The listing builds one solid part. Answer for the finished solid, in the listing's coordinates (mm). A direction names the side the tool comes from. Give positions to 0.01 mm unless a question says otherwise; leave off trailing zeros. Write each loop counter-clockwise with the first axis right and the second up, starting at its lowest first coordinate (ties: lowest second). Pieces come first, ordered by that corner, then holes. Notation, with made-up numbers: (24.25, -8.75) -> (57.25, -8.75) arc R9 ccw to (57.25, 2.25) -> close; hole circle Ø10 at (20, 31). An arc over 180 degrees is marked (long way). Put each result on its own line as item: value. Start each with the question number.
1) Flat-ended cylindrical pins translate along their axes: pin 1 Ø3.5 at (x, z) = (20.07, -1.25) entering from -Y; pin 2 Ø1.8 at (x, z) = (-8.86, -1.25) entering from +Y; pin 3 Ø7.5 at (x, y) = (11, 8) entering from +Z; pin 4 Ø1.1 at (y, z) = (13.5, 14) entering from +X. Find the tip coordinate at first contact, or state that the pin passes through.
2) A cutting plane is placed at A-A (z = 1). Write down the section's boundary in (x, y), then the cut area to 3 significant figures.
3) A cutting plane is placed at D-D (x = -11). Write down the section's boundary in (y, z).
4) Find the intervals of material crossed by line 1 along Z through (x, y) = (13.5, 10.75); line 2 along X through (y, z) = (6.5, 3); line 3 along Z through (x, y) = (20.5, 11.75), in increasing order. Write a range as from..to.
5) A cutting plane is placed at B-B (x = -1). Write down the section's boundary in (y, z).
6) For a pull along Z with two mould halves and no side action, classify faces 4 (the flat face through (6, 0, -9)), 5 (the flat face through (6, 7, 4.75)), 6 (the cylindrical face through (-7.93, 14.01, -0.66)), 7 (the flat face through (6, 8, -12.536)) as released by +Z, released by -Z, zero draft, split by the parting line, or undercut.
7) A cutting plane is placed at C-C (y = 10). Write down the section's boundary in (x, z), then the cut area to 3 significant figures.
8) For faces 1 (the flat face through (6, 7, -7.25)), 2 (the flat face through (-13, 12, 2.464)), 3 (the flat face through (-11.714, 13, -15)), determine the directions among +Z, -Z, +X, -X, +Y, -Y from which every point of the face is accessible in a straight line to the end or side of a thin tool.
from build123d import *

# Parameters (mm, degrees)
ESQUISSE1_W             = 34.285714285
ESQUISSE1_H             = 23
ESQUISSE1_W_2           = 25
ESQUISSE1_H_2           = 12
BOSS_EXTRU_1_DEPTH      = 15
ESQUISSE2_W             = 7
ESQUISSE2_H             = 8
ENL_V_MAT_EXTRU_1_DEPTH = 60
ESQUISSE3_R             = 1.1
ENL_V_MAT_EXTRU_2_DEPTH = 10
ESQUISSE4_W             = 7
ESQUISSE4_H             = 8
BOSS_EXTRU_2_DEPTH      = 20
ESQUISSE7_W             = 23
ESQUISSE7_H             = 11.477873567
ENL_V_MAT_EXTRU_3_DEPTH = 20
ESQUISSE6_R             = 1
ENL_V_MAT_EXTRU_4_DEPTH = 20


with BuildPart() as part:
    # Esquisse1 → Boss.-Extru.1 (new body)
    with BuildSketch(Plane(origin=(0, 0, 0), x_dir=(1, 0, 0), z_dir=(0, 1, 0))):
        with Locations((5.428571429, 1.035714286)):
            Rectangle(ESQUISSE1_W, ESQUISSE1_H)
        with Locations((6.142857143, 1.25)):
            Rectangle(ESQUISSE1_W_2, ESQUISSE1_H_2, mode=Mode.SUBTRACT)
    extrude(amount=BOSS_EXTRU_1_DEPTH)

    # Esquisse2 → Enlèv. mat.-Extru.1 (cut)
    with BuildSketch(Plane.ZY.offset(11.714285714)):
        with Locations((-1.035714286, 9)):
            Rectangle(ESQUISSE2_W, ESQUISSE2_H)
    extrude(amount=-ENL_V_MAT_EXTRU_1_DEPTH, mode=Mode.SUBTRACT)

    # Esquisse3 → Enlèv. mat.-Extru.2 (cut)
    with BuildSketch(Plane(origin=(0, 15, 0), x_dir=(1, 0, 0), z_dir=(0, 1, 0))):
        with Locations(Location((-8.857142857, 1.25, 0), (0, 0, 270))):
            Circle(ESQUISSE3_R)
        with Locations(Location((20.071428571, 1.25, 0), (0, 0, 270))):
            Circle(ESQUISSE3_R)
    extrude(amount=-ENL_V_MAT_EXTRU_2_DEPTH, mode=Mode.SUBTRACT)

    # Esquisse4 → Boss.-Extru.2 (add)
    with BuildSketch(Plane.ZY.offset(11.714285714)):
        Polygon((-12.535714286, 11.477873567), (-12.535714286, 0), (10.464285714, 0), (10.464285714, 11.477873567), (15.464285714, 11.477873567), (15.464285714, 15), (-17.595238813, 15), (-17.595238813, 11.477873567), align=None)
        with Locations((-1.035714286, 9)):
            Rectangle(ESQUISSE4_W, ESQUISSE4_H, mode=Mode.SUBTRACT)
    extrude(amount=BOSS_EXTRU_2_DEPTH)

    # Esquisse7 → Enlèv. mat.-Extru.3 (cut)
    with BuildSketch(Plane.ZY.offset(31.714285714)):
        with Locations((-1.035714286, 5.738936784)):
            Rectangle(ESQUISSE7_W, ESQUISSE7_H)
    extrude(amount=-ENL_V_MAT_EXTRU_3_DEPTH, mode=Mode.SUBTRACT)

    # Esquisse6 → Enlèv. mat.-Extru.4 (cut)
    with BuildSketch(Plane(origin=(0, 15, 0), x_dir=(1, 0, 0), z_dir=(0, 1, 0))):
        with Locations(Location((-25.64568933, 14.541881164, 0), (0, 0, 270))):
            Circle(ESQUISSE6_R)
        with Locations(Location((-17.64568933, 14.541881164, 0), (0, 0, 270))):
            Circle(ESQUISSE6_R)
        with Locations(Location((-25.636053252, -12.423788749, 0), (0, 0, 270))):
            Circle(ESQUISSE6_R)
        with Locations(Location((-17.636053252, -12.423788749, 0), (0, 0, 270))):
            Circle(ESQUISSE6_R)
    extrude(amount=-ENL_V_MAT_EXTRU_4_DEPTH, mode=Mode.SUBTRACT)


solid = part.part
Reply:
1. pin 1: stops at y = 0
1. pin 2: stops at y = 5
1. pin 3: stops at z = 10.46
1. pin 4: stops at x = -11.71
2. outline: (-31.71, 13) -> (-6.36, 13) -> (-6.36, 15) -> (-31.71, 15) -> close; (-11.71, 0) -> (-6.36, 0) -> (-6.36, 5) -> (-11.71, 5) -> close; (18.64, 0) -> (22.57, 0) -> (22.57, 5) -> (18.64, 5) -> close; (18.64, 13) -> (22.57, 13) -> (22.57, 15) -> (18.64, 15) -> close
2. area: 105 mm2
3. outline: (0, -12.54) -> (15, -12.54) -> (15, 10.46) -> (0, 10.46) -> close; hole (5, -4.54) -> (13, -4.54) -> (13, 2.46) -> (5, 2.46) -> close
4. line 1: z = -12.54..-7.25, 4.75..10.46
4. line 2: x = -11.71..-6.36, 18.64..22.57
4. line 3: z = -12.54..-4.54, 2.46..10.46
5. outline: (0, -12.54) -> (15, -12.54) -> (15, -7.25) -> (0, -7.25) -> close; (0, 4.75) -> (15, 4.75) -> (15, 10.46) -> (0, 10.46) -> close
6. face 4: zero draft
6. face 5: undercut
6. face 6: undercut
6. face 7: released by -Z
7. outline: (-11.71, -12.54) -> (22.57, -12.54) -> (22.57, -4.54) -> (18.64, -4.54) -> (18.64, -7.25) -> (-6.36, -7.25) -> (-6.36, -4.54) -> (-11.71, -4.54) -> close; (-11.71, 2.46) -> (-6.36, 2.46) -> (-6.36, 4.75) -> (18.64, 4.75) -> (18.64, 2.46) -> (22.57, 2.46) -> (22.57, 10.46) -> (-11.71, 10.46) -> close
7. area: 424 mm2
8. face 1: +Y, -Y
8. face 2: +X, -X
8. face 3: -Z, +X, +Y, -Y
